The drawing under review shows one solid part. Ordinate dimensions are in mm from its lowest x, y, z. A direction names the side the tool comes from. Give positions to 0.01 mm unless a question says otherwise; leave off trailing zeros. Loops run counter-clockwise (first coordinate to the right, second up) from the corner with the lowest first, then second, coordinate; pieces in that order, holes last. Notation, with made-up numbers: M 44.5,-16.5 L 99.5,-16.5 A23 cw 99.5,2.5 Z; hole C 6,68 d8. An arc over 180 degrees is marked long. Write item = value, one per line. Start each with the question number.
1. For pin 1 (8 mm diameter, centred on x = 35, z = 88, fed in from +Y); pin 2 (4 mm diameter, centred on x = 15, z = 8, fed in from +Y); pin 3 (1.5 mm diameter, centred on x = 7.5, z = 60, fed in from -Y); pin 4 (5 mm diameter, centred on x = 29.5, y = 34.5, fed in from -Z), all flat-tipped, find the tip position at first contact; note any pin that passes through.
2. We need section A-A on x = 25. Give the boundary of the cut face in (y, z).
3. We need section C-C on x = 15. Give the boundary of the cut face in (y, z).
4. Wall thickness on line 1 along Y through (x, z) = (25, 102.05); line 2 along Z through (x, y) = (28.5, 32); line 3 along Y through (x, z) = (31, 60): over which ranges is each line inside the solid? List them lowest first. Write a range as from..to.
5. For the marked faces 1 and 2, list the 3-axis set-ups (+Z, -Z, +X, -X, +Y, -Y) from which the entire face can be reached by the end or side of a thin tool; tool diameter is ignored.
6. We need section B-B on y = 58. Give the boundary of the cut face in (x, z).
7. We need section D-D on z = 15. Give the boundary of the cut face in (x, y).
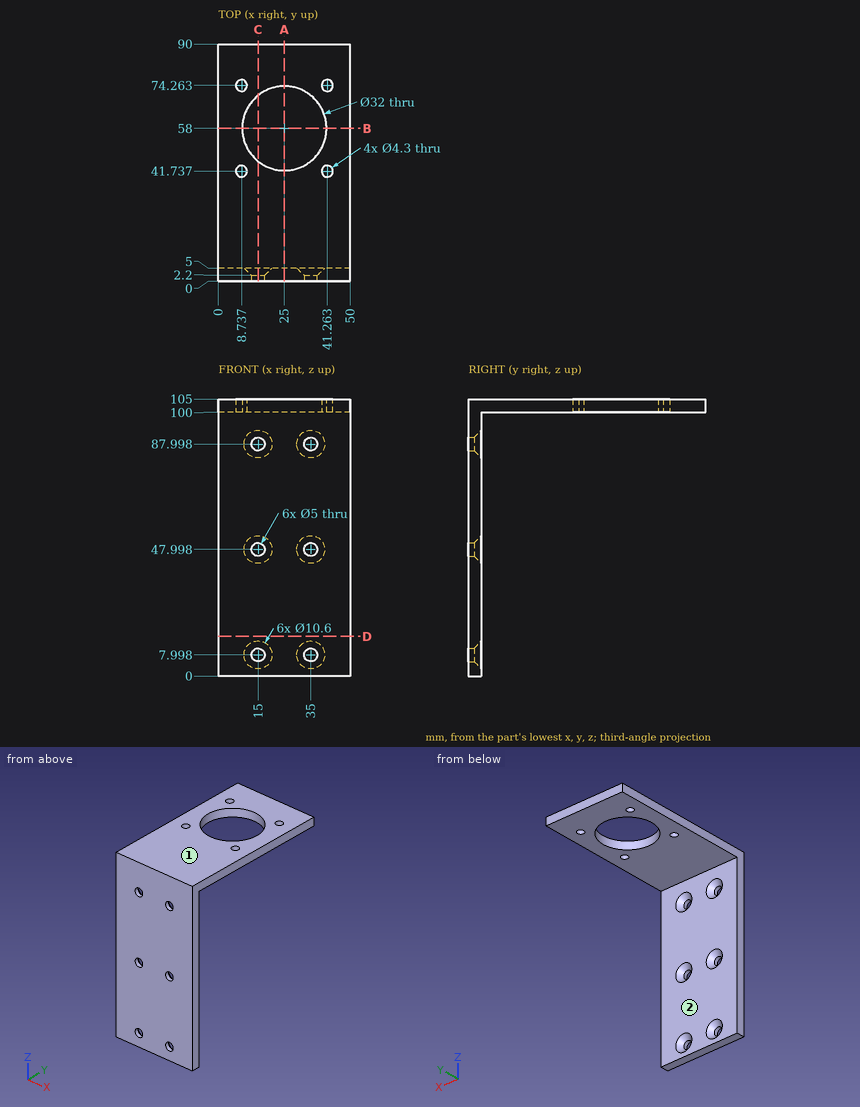
Final values:
q1.pin_1 = 3.7
q1.pin_2 = through
q1.pin_3 = 0
q1.pin_4 = 100
q2.outline = M 0,0 L 5,0 L 5,100 L 42,100 L 42,105 L 0,105 Z; M 74,100 L 90,100 L 90,105 L 74,105 Z
q3.outline = M 0,0 L 5,0 L 5,2.7 L 2.2,5.5 L 0,5.5 Z; M 0,10.5 L 2.2,10.5 L 5,13.3 L 5,42.7 L 2.2,45.5 L 0,45.5 Z; M 0,50.5 L 2.2,50.5 L 5,53.3 L 5,82.7 L 2.2,85.5 L 0,85.5 Z; M 0,90.5 L 2.2,90.5 L 5,93.3 L 5,100 L 45.51,100 L 45.51,105 L 0,105 Z; M 70.49,100 L 90,100 L 90,105 L 70.49,105 Z
q4.line_1 = 0..42, 74..90
q4.line_2 = 100..105
q4.line_3 = 0..5
q5.face_1 = +Z, +X, -X, +Y, -Y
q5.face_2 = -Z, +X, -X, +Y
q6.outline = M 0,100 L 9,100 L 9,105 L 0,105 Z; M 41,100 L 50,100 L 50,105 L 41,105 Z
q7.outline = M 0,0 L 50,0 L 50,5 L 0,5 Z
